Autodesk Inventor part; units mm, degrees
ref_plane "YZ Plane" through (0, 0, 0) normal (1, 0, 0) x (0, 1, 0)
ref_plane "XZ Plane" through (0, 0, 0) normal (0, 1, 0) x (-1, 0, 0)
ref_plane "XY Plane" through (0, 0, 0) normal (0, 0, 1) x (1, 0, 0)
sketch "スケッチ12" plane through (0, 0, 0) normal (0, 0, 1) x (1, 0, 0)
  circle A0 centre (0, 0) radius 27.5
  circle A1 centre (0, 0) radius 15
  line L0 (-27.5, 0) -> (27.5, 0)
  line L1 (-27.5, 0) -> (-9.3015, 50)
  line L2 (-9.3015, 50) -> (9.3015, 50)
  line L3 (9.3015, 50) -> (27.5, 0)
  circle A2 centre (0, 40) radius 4
  line L4 (9.3015, 50) -> (-27.5, 0)
  line L5 (-9.3015, 50) -> (27.5, 0)
  point P0 (21.0662, 17.6767)
  point P1 (-21.0662, 17.6767)
  point P2 (0, 51.9615)
  point P3 (8.174, 26.2571)
  point P4 (-8.174, 26.2571)
  point P5 (-2.2669, 48.0351)
  point P6 (2.2669, 48.0351)
  point P7 (0, 37.3626)
  point P8 (-15, 0)
  point P9 (15, 0)
  dimension "d5" = 55
  dimension "d6" = 30
  dimension "d10" = 70
  dimension "d11" = 70
  dimension "d12" = 50
  dimension "d13" = 40
  dimension "d14" = 8
  dimension "d47" = 0
extrude "押し出し2" add sketch "スケッチ12" along normal blind 5 contours L0 A1 A0 | L4 A0 L5 L0 A1 | A0 L1 | L1 A0 L4 | L3 A0 | L5 A0 L3 | L1 L5 A2 L4 A0 | L4 A2 L5 A0 | A0 L5 A2 L4 L3 | L2 L4 A2 L5
sketch "スケッチ13" plane through (0, 0, 5) normal (0, 0, 1) x (1, 0, 0)
  circle A0 centre (0, 0) radius 17.5
  circle A1 centre (0, 0) radius 25
  circle A2 centre (0, 0) radius 21.25
  line L0 (0, 0) -> (-18.638, 32.282)
  line L1 (-18.638, 32.282) -> (0, 0)
  line L2 (0, 0) -> (-17.2844, -29.9374)
  line L3 (0, 0) -> (-56.8729, 0)
  line L4 (0, 0) -> (-31.7394, -18.3248)
  line L5 (0, 0) -> (-33.3883, 19.2767)
  line L6 (0, 0) -> (0, -31.9785)
  line L7 (0, 0) -> (-25.7143, 25.7143)
  line L8 (0, 0) -> (-33.0547, 8.857)
  line L9 (0, 0) -> (-32.621, -8.7408)
  line L10 (0, 0) -> (-23.652, -23.652)
  point P0 (-18.403, 10.625)
  point P1 (-21.25, 0)
  point P2 (-18.403, -10.625)
  point P3 (-10.625, -18.403)
  point P4 (0, -21.25)
  point P5 (-16.5273, 4.4285)
  point P6 (-15.026, 15.026)
  point P7 (-20.5259, 5.4999)
  point P8 (-20.5259, -5.4999)
  point P9 (-15.026, -15.026)
  dimension "d19" = 42.5
  dimension "d17" = 35
  dimension "d18" = 50
  dimension "d20" = 60
  dimension "d21" = 60
  dimension "d22" = 30
  dimension "d23" = 30
  dimension "d31" = 150
  dimension "d32" = 15
  dimension "d34" = 15
  dimension "d35" = 15
  dimension "d36" = 15
hole "穴1" at (-15.026, 15.026, 5) at (-20.5259, 5.4999, 5) at (-20.5259, -5.4999, 5) at (-15.026, -15.026, 5) direction (0, 0, -1) diameter 3 end through all
sketch "スケッチ14" plane through (0, 0, 5) normal (0, 0, 1) x (1, 0, 0)
  circle A0 centre (-15.026, 15.026) radius 1.5
  circle A1 centre (-15.026, 15.026) radius 3
  circle A2 centre (-20.5259, 5.4999) radius 1.5
  circle A3 centre (-20.5259, 5.4999) radius 3
  circle A4 centre (-20.5259, -5.4999) radius 1.5
  circle A5 centre (-20.5259, -5.4999) radius 3
  circle A6 centre (-15.026, -15.026) radius 1.5
  circle A7 centre (-15.026, -15.026) radius 3
  point P0 (0, 0)
  dimension "d40" = 6
  dimension "d41" = 6
  dimension "d42" = 6
  dimension "d43" = 6
extrude "押し出し3" cut sketch "スケッチ14" against normal blind 2 contours A0 | A1 | A2 | A3 | A4 | A5 | A6 | A7
fillet "フィレット3" radius 13.5 2 edges at (9.3015, 50, 2.5) (-9.3015, 50, 2.5)
equation "\"d10\" = d11"
equation "\"d35\" = d34"
equation "\"d36\" = d35"
equation "\"d41\" = d40"
equation "\"d42\" = d41"
equation "\"d43\" = d42"
properties part number "legparts_04(seven)" material "ABS プラスチック"
Part model, mm, in its own coordinate system. A direction names the side the tool comes from. Coordinates: 2 decimals unless noted, no trailing zeros. Loops run counter-clockwise (first coordinate to the right, second up) from the corner with the lowest first, then second, coordinate; pieces in that order, holes last. Notation, with made-up numbers: M 76.25,32 L 132.25,32 A18 cw 132.25,40 Z; hole C -9.5,36 d8. An arc over 180 degrees is marked long. Use a Markdown table: item, result. Add a question column.
Q1. Pin check, flat tips, straight feed: P1, Ø5, axis at x = -20.53, y = 5.5, coming from the +Z side; P2, Ø5, axis at x = -19, y = -6.5, coming from the +Z side; P3, Ø2.5, axis at x = -15.026, y = 15.026, coming from the -Z side. Stop position of each tip, or through.
Q2. Mould opens along Y. For faces 3 (the flat face through (0, 20, 5)), 4 (the flat face through (16.8, 29.4, 2.5)), 5 (the cylindrical face through (-17.755, 4.351, 4.014)), 6 (the flat face through (-13.7, -16.3, 3)) say: +Y half, -Y half, draft (parallel to the pull), parting line (faces both ways), or undercut.
Q3. Probe L1, parallel to Y at x = 0, z = 2.9; L2, parallel to X at y = 26, z = 3.4; L3, parallel to X at y = 0, z = 2.45. List the from-to ranges inside material, lowest first.
Q4. Cut at A-A (y = 0). Write the cut outline in (x, z).
Q5. Cut at B-B (x = 0). Give the number of separate pieces and of enclosed holes in the cut face, and give its area (3 significant figures).
Q6. Cut at C-C (y = 39). Write the cut outline in (x, z), and give its area (3 significant figures).
Q7. Which spindle directions (+Z, -Z, +X, -X, +Y, -Y) get a long thin tool onto all of the face, cutting with end or side? Do faces 1 (the flat face through (-19, -7, 3)), 2 (the cylindrical face through (-14.45, -16.41, 1.48)). Say none if no direction does.
Worked out:
| question | item | result |
|---|---|---|
| 1 | P1 | stops at z = 3 |
| 1 | P2 | stops at z = 5 |
| 1 | P3 | passes through |
| 2 | face 3 | draft |
| 2 | face 4 | +Y half |
| 2 | face 5 | undercut |
| 2 | face 6 | undercut |
| 3 | L1 | y = -27.5 to -15, 15 to 36, 44 to 49.58 |
| 3 | L2 | x = -18.04 to 18.04 |
| 3 | L3 | x = -27.5 to -15, 15 to 27.5 |
| 4 | outline | M -27.5,0 L -15,0 L -15,5 L -27.5,5 Z; M 15,0 L 27.5,0 L 27.5,5 L 15,5 Z |
| 5 | separate pieces | 3 |
| 5 | enclosed holes | 0 |
| 5 | area | 195 mm2 |
| 6 | outline | M -13.31,0 L -3.87,0 L -3.87,5 L -13.31,5 Z; M 3.87,0 L 13.31,0 L 13.31,5 L 3.87,5 Z |
| 6 | area | 94.3 mm2 |
| 7 | face 1 | +Z |
| 7 | face 2 | +Z, -Z |
